Design review of the part built by this model. Coordinates are the model's own, in mm. Face numbers are marked on the shaded views. A direction names the side the tool comes from. Coordinates: 2 decimals unless noted, no trailing zeros. Write each loop counter-clockwise with the first axis right and the second up, starting at its lowest first coordinate (ties: lowest second). Pieces come first, ordered by that corner, then holes.
Q1. Machinability: for the marked faces 1, 2 and 3, which of the approach directions +Z, -Z, +X, -X, +Y, -Y give a long, thin tool a straight path to every point of the face, cutting with its end or side? Answer none if there is none.
Q2. Take a section at D-D (z = -47). Give the boundary of the cut face in (x, y), and give its area (3 significant figures).
Q3. Take a section at B-B (y = -14.5). Give the boundary of the cut face in (x, z), and give its area (3 significant figures).
Q4. Mouldability with a two-part tool opening along Z and no side actions: class the marked faces 4, 5, 6 and 7 as pulls with the +Z half, pulls with the -Z half, needs draft (parallel to the pull), parting line crosses it, or undercut.
Q5. Take a section at A-A (z = -34). Give the boundary of the cut face in (x, y).
Q6. For probe 1 along Z at (x, y) = (-19.5, -2.5); probe 2 along Z at (x, y) = (5.5, -10.5); probe 3 along X at (y, z) = (-7, -35.5), list the stretches that pass through material, from the lowest coordinate up.
Q7. Take a section at C-C (x = 1). Give the boundary of the cut face in (y, z).
Q8. Insertion check: pin 1 (4 mm diameter, centred on x = -14.5, z = -28, fed in from -Y); pin 2 (8 mm diameter, centred on x = 17.5, z = 6.5, fed in from -Y). Each pin has a flat end and moves straight along its axis. Give the tip position at first contact, or say it passes through.
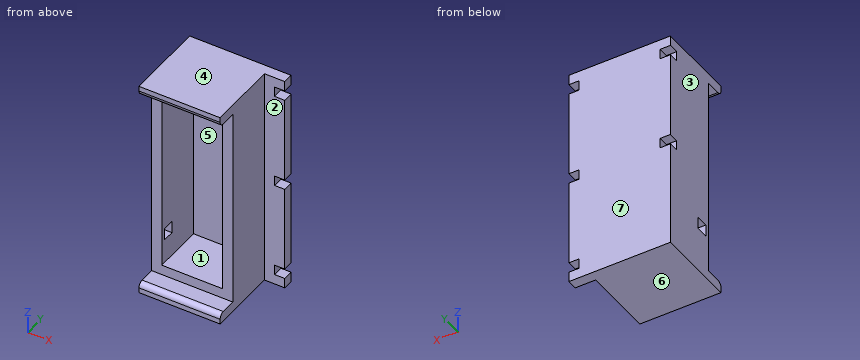
```python
from build123d import *

# Parameters (mm, degrees)
SKETCH2_W           = 40
SKETCH2_H           = 5
SKETCH2_W_2         = 5
SKETCH2_H_2         = 100
BOSS_EXTRUDE1_DEPTH = 30
SKETCH3_W           = 3
SKETCH3_H           = 3
CUT_EXTRUDE1_DEPTH  = 5
SKETCH2_4_W         = 40
SKETCH2_4_H         = 100
BOSS_EXTRUDE2_DEPTH = 5
CUT_EXTRUDE2_DEPTH  = 25
BOSS_EXTRUDE3_DEPTH = 25
SKETCH10_W          = 40
SKETCH10_H          = 5
BOSS_EXTRUDE4_DEPTH = 35
SKETCH11_W          = 5
SKETCH11_H          = 5
CUT_EXTRUDE5_DEPTH  = 6
SKETCH11_4_W        = 5
SKETCH11_4_H        = 5
CUT_EXTRUDE6_DEPTH  = 4.99
FILLET1_R           = 2.5


with BuildPart() as part:
    # Sketch2 → Boss-Extrude1 (new body)
    with BuildSketch(Plane(origin=(0, 0, 0), x_dir=(1, 0, 0), z_dir=(0, 1, 0))):
        Polygon((-22.5, 60), (-22.5, -50), (-17.5, -50), (-17.5, -45), (-17.5, 55), (-17.5, 60), align=None)
        with Locations((2.5, 57.5)):
            Rectangle(SKETCH2_W, SKETCH2_H)
        with Locations((25, 57.5)):
            Rectangle(SKETCH2_W_2, SKETCH2_H)
        with Locations((25, 5)):
            Rectangle(SKETCH2_W_2, SKETCH2_H_2)
        with Locations((25, -47.5)):
            Rectangle(SKETCH2_W_2, SKETCH2_H)
        with Locations((2.5, -47.5)):
            Rectangle(SKETCH2_W, SKETCH2_H)
    extrude(amount=-BOSS_EXTRUDE1_DEPTH)

    # Sketch3 → Cut-Extrude1 (cut)
    with BuildSketch(Plane.ZY.offset(22.5)):
        Polygon((-35, -25), (-35, -28), (-32, -28), (-32, -22), (-38, -22), (-38, -25), align=None)
        with Locations((-36.5, -26.5)):
            Rectangle(SKETCH3_W, SKETCH3_H)
    extrude(amount=-CUT_EXTRUDE1_DEPTH, mode=Mode.SUBTRACT)

    # Sketch2_4 → Boss-Extrude2 (add)
    with BuildSketch(Plane(origin=(0, 0, 0), x_dir=(1, 0, 0), z_dir=(0, 1, 0))):
        with Locations((2.5, 5)):
            Rectangle(SKETCH2_4_W, SKETCH2_4_H)
    extrude(amount=-BOSS_EXTRUDE2_DEPTH)

    # Sketch5 → Cut-Extrude2 (cut)
    with BuildSketch(Plane.XZ.offset(30)):
        Polygon((27.5, 50), (-22.5, 50), (-22.5, 45), (-17.5, 45), (17.5, 45), (22.5, 45), (22.5, -55), (17.5, -55), (-17.5, -55), (-22.5, -55), (-22.5, -60), (27.5, -60), align=None)
    extrude(amount=-CUT_EXTRUDE2_DEPTH, mode=Mode.SUBTRACT)

    # Sketch5_3 → Boss-Extrude3 (add)
    with BuildSketch(Plane.XZ.offset(30)):
        Polygon((17.5, 45), (-17.5, 45), (-17.5, 40), (12.5, 40), (12.5, -50), (-17.5, -50), (-17.5, -55), (17.5, -55), align=None)
    extrude(amount=-BOSS_EXTRUDE3_DEPTH)

    # Sketch10 → Boss-Extrude4 (add)
    with BuildSketch(Plane.XZ.offset(5)):
        with Locations((-2.5, 47.5)):
            Rectangle(SKETCH10_W, SKETCH10_H)
        with Locations((-2.5, -57.5)):
            Rectangle(SKETCH10_W, SKETCH10_H)
    extrude(amount=BOSS_EXTRUDE4_DEPTH)

    # Sketch11 → Cut-Extrude5 (cut)
    with BuildSketch(Plane(origin=(0, 0, 0), x_dir=(1, 0, 0), z_dir=(0, 1, 0))):
        with Locations((25, 52.5)):
            Rectangle(SKETCH11_W, SKETCH11_H)
        Polygon((27.5, 7.5), (22.5, 7.5), (22.5, 5), (22.5, 2.5), (27.5, 2.5), (27.5, 5), align=None)
        Polygon((27.5, -45), (27.5, -40), (24, -40), (23.5, -40), (22.5, -40), (22.5, -41), (22.5, -41.5), (22.5, -45), align=None)
    extrude(amount=-CUT_EXTRUDE5_DEPTH, mode=Mode.SUBTRACT)

    # Sketch11_4 → Cut-Extrude6 (cut)
    with BuildSketch(Plane(origin=(0, 0, 0), x_dir=(1, 0, 0), z_dir=(0, 1, 0))):
        Polygon((-17.5, 7.5), (-22.5, 7.5), (-22.5, 5), (-22.5, 2.5), (-17.5, 2.5), align=None)
        with Locations((-20, -42.5)):
            Rectangle(SKETCH11_4_W, SKETCH11_4_H)
    extrude(amount=-CUT_EXTRUDE6_DEPTH, mode=Mode.SUBTRACT)

    # Fillet1
    fillet1_edges = [part.edges().sort_by_distance(p)[0] for p in [
        (-2.5, -40, 45),
        (-2.5, -40, -55),
    ]]
    fillet(fillet1_edges, radius=FILLET1_R)


solid = part.part
```
Response:
1. face 1: -Y
1. face 2: +Z, -Z, +X, -Y
1. face 3: +Z, -Z, -X, +Y, -Y
2. outline: (-22.5, -30) - (-17.5, -30) - (-17.5, -5) - (12.5, -5) - (12.5, -30) - (17.5, -30) - (17.5, -5) - (27.5, -5) - (27.5, 0) - (-22.5, 0) - close
2. area: 500 mm2
3. outline: (-22.5, -60) - (17.5, -60) - (17.5, 50) - (-22.5, 50) - close; hole (-17.5, -50) - (12.5, -50) - (12.5, 40) - (-17.5, 40) - close
3. area: 1,700 mm2
4. face 4: pulls with the +Z half
4. face 5: undercut
4. face 6: pulls with the -Z half
4. face 7: needs draft
5. outline: (-22.5, -30) - (-17.5, -30) - (-17.5, -28) - (-22.5, -28) - close; (-22.5, -22) - (-17.5, -22) - (-17.5, -5) - (12.5, -5) - (12.5, -30) - (17.5, -30) - (17.5, -5) - (27.5, -5) - (27.5, 0) - (-22.5, 0) - close
6. probe 1: z = -60 to -7.5, -2.5 to 40, 45 to 50
6. probe 2: z = -60 to -50, 40 to 50
6. probe 3: x = -22.5 to -17.5, 12.5 to 17.5
7. outline: (-40, -60) - (0, -60) - (0, 50) - (-40, 50) - (-40, 47.5) arc R2.5 ccw to (-37.5, 45) - (-30, 45) - (-30, 40) - (-5, 40) - (-5, -50) - (-30, -50) - (-30, -55) - (-37.5, -55) arc R2.5 ccw to (-40, -57.5) - close
8. pin 1: stops at y = -5
8. pin 2: stops at y = -30
